Could you check a few things on this model? Use its own coordinates, in mm. Face numbers are marked on the shaded views. A direction names the side the tool comes from. Coordinates: 2 decimals unless noted, no trailing zeros. Loops run counter-clockwise (first coordinate to the right, second up) from the corner with the lowest first, then second, coordinate; pieces in that order, holes last. Notation, with made-up numbers: (-23, 3) -> (24, 3) arc R10 ccw to (24, 7) -> close; hole circle Ø5 at (84.25, -30.5). An arc over 180 degrees is marked (long way). One line per question, with ' | ' between items.
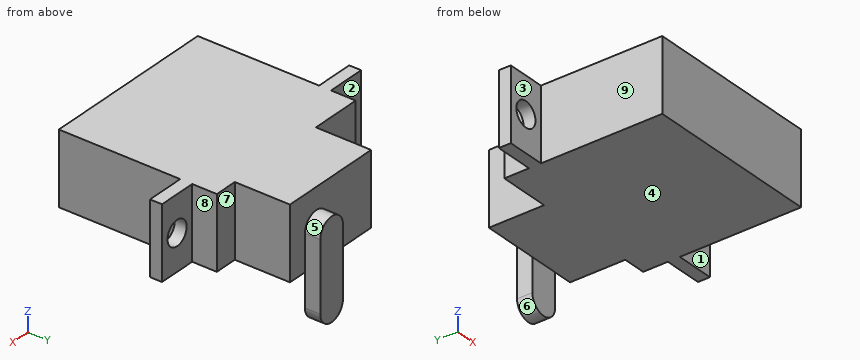
from build123d import *

# Parameters (mm, degrees)
SKETCH3_W           = 29.5148
SKETCH3_H           = 11.938
BOSS_EXTRUDE1_DEPTH = 26.162
SKETCH4_W           = 11.938
SKETCH4_H           = 1.9812
BOSS_EXTRUDE2_DEPTH = 6.4008
SKETCH5_R           = 2.032
CUT_EXTRUDE1_DEPTH  = 6.4008
SKETCH6_W           = 17.2466
SKETCH6_H           = 11.938
BOSS_EXTRUDE3_DEPTH = 9.144
BOSS_EXTRUDE4_DEPTH = 2.54


with BuildPart() as part:
    # Sketch3 → Boss-Extrude1 (new body)
    with BuildSketch(Plane(origin=(0, 0, 0), x_dir=(1, 0, 0), z_dir=(0, 1, 0))):
        with Locations((14.7574, -5.969)):
            Rectangle(SKETCH3_W, SKETCH3_H)
    extrude(amount=BOSS_EXTRUDE1_DEPTH)

    # Sketch4 → Boss-Extrude2 (add)
    with BuildSketch(Plane(origin=(29.5148, 0, 0), x_dir=(0, 0, -1), z_dir=(1, 0, 0))):
        with Locations((-5.969, 21.082)):
            Rectangle(SKETCH4_W, SKETCH4_H)
    boss_extrude2 = extrude(amount=BOSS_EXTRUDE2_DEPTH)

    # Mirror1: Boss-Extrude2 across plane
    add(boss_extrude2.mirror(Plane(origin=(14.7574, 0, 0), x_dir=(0, 0, 1), z_dir=(1, 0, 0))))

    # Sketch5 → Cut-Extrude1 (cut)
    with BuildSketch(Plane(origin=(0, 22.0726, 0), x_dir=(1, 0, 0), z_dir=(0, 1, 0))):
        with Locations((32.7152, -5.969)):
            Circle(SKETCH5_R)
    cut_extrude1 = extrude(amount=-CUT_EXTRUDE1_DEPTH, mode=Mode.SUBTRACT)

    # Mirror2: Cut-Extrude1 across plane
    add(cut_extrude1.mirror(Plane(origin=(14.7574, 0, 0), x_dir=(0, 0, 1), z_dir=(1, 0, 0))), mode=Mode.SUBTRACT)

    # Sketch6 → Boss-Extrude3 (add)
    with BuildSketch(Plane(origin=(0, 26.162, 0), x_dir=(1, 0, 0), z_dir=(0, 1, 0))):
        with Locations((17.0815, -5.969)):
            Rectangle(SKETCH6_W, SKETCH6_H)
    extrude(amount=BOSS_EXTRUDE3_DEPTH)

    # Sketch7 → Boss-Extrude4 (add)
    with BuildSketch(Plane(origin=(0, 35.306, 0), x_dir=(1, 0, 0), z_dir=(0, 1, 0))):
        with BuildLine():
            Line((17.7038, -5.969), (17.7038, 5.461))
            ThreePointArc((17.7038, 5.461), (20.1168, 7.874), (22.5298, 5.461))
            Line((22.5298, 5.461), (22.5298, -5.969))
            ThreePointArc((22.5298, -5.969), (20.1168, -8.382), (17.7038, -5.969))
        make_face()
    extrude(amount=BOSS_EXTRUDE4_DEPTH)


solid = part.part
1) I'm going to push flat-ended pins straight in: pin 1 Ø10 at (y, z) = (31.5, 10) entering from -X; pin 2 Ø4.5 at (y, z) = (24.5, 9) entering from -X; pin 3 Ø2 at (y, z) = (24, 3) entering from +X. Where does each tip first touch, or does it pass through?
Data:
pin 1: x = 8.46 | pin 2: x = 0 | pin 3: x = 29.51
2) I need wall thicknesses on line 1 along Z through (x, y) = (17.5, 32); line 2 along Y through (x, z) = (32.5, 9); line 3 along X through (y, z) = (15.5, 6.5). Which ranges of each line are inside material? Lowest first, please. Write a range as from..to.
Data:
line 1: 0..11.94 | line 2: 20.09..22.07 | line 3: 0..29.51
3) On a 3-axis mill with a long thin cutter (end or side, diameter ignored), from which of +Z, -Z, +X, -X, +Y, -Y can I reach the whole of each face in a straight line? I mean the marked faces 1, 2, 3, 4 and 5. Say none if no direction works.
Data:
face 1: +Z, -Z, +X, -Y | face 2: +Z, -Z, -X, +Y | face 3: +Z, -Z, -X, -Y | face 4: -Z, +X, -X, -Y | face 5: +Z, +Y
4) We'd pull the mould along X, two halves only. Please class the marked faces 6, 7, 8 and 9: pulls with the +X half, pulls with the -X half, needs draft (parallel to the pull), parting line crosses it, or undercut.
Data:
face 6: parting line crosses it | face 7: needs draft | face 8: pulls with the +X half | face 9: pulls with the -X half
5) If we section it at D-D on y = 11: Please give me the cut outline in (x, z), and give its area (3 significant figures).
Data:
outline: (0, 0) -> (29.51, 0) -> (29.51, 11.94) -> (0, 11.94) -> close | area: 352 mm²
6) If we section it at A-A on z = 0.5: Please give me the cut outline in (x, y), and give its area (3 significant figures).
Data:
outline: (-6.4, 20.09) -> (0, 20.09) -> (0, 0) -> (29.51, 0) -> (29.51, 20.09) -> (35.92, 20.09) -> (35.92, 22.07) -> (29.51, 22.07) -> (29.51, 26.16) -> (25.7, 26.16) -> (25.7, 35.31) -> (22.53, 35.31) -> (22.53, 37.85) -> (17.7, 37.85) -> (17.7, 35.31) -> (8.46, 35.31) -> (8.46, 26.16) -> (0, 26.16) -> (0, 22.07) -> (-6.4, 22.07) -> close | area: 967 mm²
7) If we section it at C-C on x = -3: Please give me the cut outline in (y, z), and give its area (3 significant figures).
Data:
outline: (20.09, 0) -> (22.07, 0) -> (22.07, 3.95) -> (20.09, 3.95) -> close; (20.09, 7.99) -> (22.07, 7.99) -> (22.07, 11.94) -> (20.09, 11.94) -> close | area: 15.6 mm²
8) If we section it at B-B on x = 20.5: Please give me the cut outline in (y, z).
Data:
outline: (0, 0) -> (35.31, 0) -> (35.31, -7.84) -> (37.85, -7.84) -> (37.85, 8.35) -> (35.31, 8.35) -> (35.31, 11.94) -> (0, 11.94) -> close
